Can you work these out from the model? Positions are in its coordinate system, mm. Face numbers are marked on the shaded views. A direction names the side the tool comes from. Give positions to 0.01 mm unless a question says otherwise; leave off trailing zeros. Order: outer loops, then holes, each group sorted by start corner. A loop starts at its lowest first (then second) coordinate and runs counter-clockwise, first axis right, second up. Notation, with made-up numbers: (25, -15) - (48, -15) arc R32 cw to (48, 20) - close; hole circle Ø6 at (61.25, -15). An arc over 180 degrees is marked (long way). Write each question's results on one line, items separated by ' | '. Start each with the question number.
Autodesk Fusion 360 part; units mm, degrees
sketch "Sketch1" plane through (0, 0, 0) normal (0, 1, 0) x (1, 0, 0) in component "ChargerSpacer"
  arc A0 (-5.8311, -8.732) -> (-5.8573, 8.7145) centre (0, 0) cw
  arc A1 (-4.6183, -9.4298) -> (-5.8311, -8.732) centre (-5.2363, -9.1011) cw
  line L0 (-20, 3.982) -> (0, 3.982)
  arc A2 (10.4756, 0.7154) -> (10.4777, -0.6839) centre (10.5, 0.0158) cw
  arc A3 (-4.6466, 9.4159) -> (10.4756, 0.7154) centre (0, 0) cw
  arc A4 (10.4777, -0.6839) -> (-4.6183, -9.4298) centre (0, 0) cw
  arc A5 (-5.8573, 8.7145) -> (-4.6466, 9.4159) centre (-5.2637, 9.0854) cw
  line L1 (-20, -4.0237) -> (-20, 3.982)
  circle A6 centre (0, 0) radius 8
  line L2 (0, 3.982) -> (0, -4.0237)
  line L3 (0, -4.0237) -> (-20, -4.0237)
  circle A7 centre (0, 0) radius 5
  circle A8 centre (0, 0) radius 3.75
  dimension "d8" = 10
  dimension "d9" = 7.5
extrude "Extrude8" add sketch "Sketch1" along normal blind 27 contours A0 A1 L0 A2 A3 A4 A5 A6 L3 | A0 L0 A6 L3 | L0 A6 L3 A7 | L0 A6 L3 A7 | L0 L2 L3 A7 A8 | L0 L2 L3 A7 A8 in component "ChargerSpacer"
sketch "Sketch2" plane through (0, 27, 0) normal (0, 1, 0) x (-1, 0, 0) in component "ChargerSpacer"
  circle A0 centre (0, 0) radius 4
  line L0 (6.35, 6.35) -> (-6.35, 6.35)
  line L1 (-6.35, 6.35) -> (-6.35, -6.35)
  line L2 (-6.35, -6.35) -> (6.35, -6.35)
  line L3 (6.35, -6.35) -> (6.35, 6.35)
  line L4 (6.35, 6.35) -> (-6.35, -6.35) construction
  line L5 (-6.35, 6.35) -> (6.35, -6.35) construction
  line L6 (6.35, 6.35) -> (19.35, 6.35)
  line L7 (19.35, 6.35) -> (19.35, -6.35)
  line L8 (19.35, -6.35) -> (6.35, -6.35)
  line L9 (6.35, -6.35) -> (6.35, 6.35)
  circle A1 centre (0, 0) radius 6.35
  line L10 (12.5, -3.5) -> (-12.5, -3.5)
  line L11 (-12.5, -3.5) -> (-12.5, 3.5)
  line L12 (-12.5, 3.5) -> (12.5, 3.5)
  line L13 (12.5, 3.5) -> (12.5, -3.5)
  line L14 (12.5, -3.5) -> (-12.5, 3.5) construction
  line L15 (-12.5, -3.5) -> (12.5, 3.5) construction
  arc A2 (5.8573, -8.7145) -> (5.8311, 8.732) centre (0, 0) ccw
  arc A3 (5.8311, 8.732) -> (4.6183, 9.4298) centre (5.2363, 9.1011) ccw
  arc A4 (4.6183, 9.4298) -> (-10.4777, 0.6839) centre (0, 0) ccw
  arc A5 (-10.4777, 0.6839) -> (-10.4756, -0.7154) centre (-10.5, -0.0158) ccw
  arc A6 (-10.4756, -0.7154) -> (4.6466, -9.4159) centre (0, 0) ccw
  arc A7 (4.6466, -9.4159) -> (5.8573, -8.7145) centre (5.2637, -9.0854) ccw
  circle A8 centre (0, 0) radius 3.75
  dimension "d18" = 12.7
  dimension "d19" = 12.7
  dimension "d20" = 13
  dimension "d21" = 12.7
  dimension "d22" = 12.7
  dimension "d27" = 25
  dimension "d28" = 7
extrude "Extrude9" cut sketch "Sketch1" along normal blind 4 contours L0 L2 L3 A7 A8 | L0 L2 L3 A7 A8 in component "ChargerSpacer"
extrude "Extrude10" add sketch "Sketch2" along normal blind 10 contours L0 L1 L6 L12 A2 A3 A4 | L3 L6 L9 L12 A2 | L1 L2 L8 L10 A2 A6 A7 | L3 L8 L9 L10 A2 | L1 L10 L12 A4 A5 A6 in component "ChargerSpacer"
extrude "Extrude11" cut sketch "Sketch2" against normal blind 17 contours A0 L10 L12 A8 | A0 A1 L10 L12 | A0 L12 A8 | A0 A1 L12 | A0 A1 L10 | A0 L10 A8 | A0 L10 L12 A8 | A0 A1 L10 L12 | L3 L9 A1 L12 | L3 L9 A1 L10 | L3 L9 L10 L12 A2 in component "ChargerSpacer"
fillet "Fillet1" radius 3 2 edges at (-7.5989, 10, -3.5) (-7.5989, 10, 3.5) in component "ChargerSpacer"
chamfer "Chamfer1" distance 0.5 angle 45 5 edges at (-6.35, 37, -4.925) (0, 37, -6.35) (-6.35, 37, 4.925) (0, 37, 6.35) (6.35, 37, 0) in component "ChargerSpacer"
component "ChargerSpacer" placed x (1, 0, 0) y (0, 1, 0) z (0, 0, 1) at (0, 0, 0)
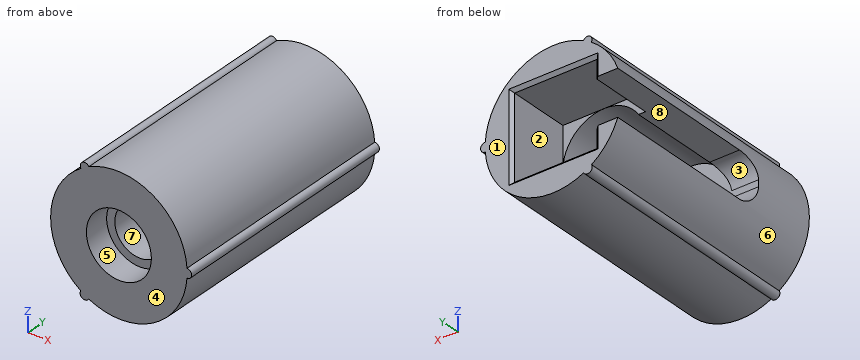
Q1. If we section it at B-B (y = 4.5): Please give me the cut outline in (x, z).
Q2. Thinking about a two-plate mould opening in X: for the marked faces 6, 7 and 8, which applies, released by +X, released by -X, zero draft, split by the parting line, or undercut?
Q3. If I drill on probe 1 along Z at (x, y) = (0, 7.8); probe 2 along Z at (x, y) = (0, 3.15); probe 3 along Y at (x, z) = (-1.5, 5.25), over which ranges is the centre line in solid material (lowest first)? Write a range as from..to.
Q4. If we section it at C-C (y = 21.5): Please give me the cut outline in (x, z).
Q5. If we section it at D-D (x = -8.75): Please give me the cut outline in (y, z).
Q6. Which directions (+Z, -Z, +X, -X, +Y, -Y) give clear straight access to the entire face, cutting with the end or side of a thin tool? Please do the marked faces 1, 2, 3, 4 and 5.
Q7. If we section it at A-A (z = -2): Please give me the cut outline in (x, y), plus the area to 3 significant figures.
Q8. Will these pins go through, and if not, where does the flat tip stop? P1, Ø3, axis at x = -4.5, z = -5, coming from the +Y side; P2, Ø0.9, axis at y = 33, z = -5, coming from the +X side; P3, Ø2, axis at x = 9, y = 30.5, coming from the +Z side; P4, Ø7.5, axis at x = -0.5, y = 31, coming from the +Z side.
Findings below:
1) outline: (-5.86, -8.71) arc R0.7 ccw (long way) to (-4.65, -9.42) arc R10.5 ccw to (10.48, -0.72) arc R0.7 ccw (long way) to (10.48, 0.68) arc R10.5 ccw to (-4.62, 9.43) arc R0.7 ccw (long way) to (-5.83, 8.73) arc R10.5 ccw to start; hole circle Ø7.5 at (0, 0)
2) face 6: released by -X | face 7: undercut | face 8: zero draft
3) probe 1: z = -10.5..-3.75, 3.75..10.5 | probe 2: z = -10.5..-5, 5..10.5 | probe 3: y = 0..10
4) outline: (-9.9, -3.5) arc R10.5 ccw to (-5.86, -8.71) arc R0.7 ccw (long way) to (-4.65, -9.42) arc R10.5 ccw to (10.48, -0.72) arc R0.7 ccw (long way) to (10.48, 0.68) arc R10.5 ccw to (-4.62, 9.43) arc R0.7 ccw (long way) to (-5.83, 8.73) arc R10.5 ccw to (-9.9, 3.5) - (-5.3, 3.5) arc R6.35 cw (long way) to (-5.3, -3.5) - close
5) outline: (0, -5.8) - (37, -5.8) - (37, -3.5) - (13, -3.5) arc R3 cw to (10, -0.5) - (10, 0.5) arc R3 cw to (13, 3.5) - (37, 3.5) - (37, 5.8) - (0, 5.8) - close
6) face 1: +Z, -Z, +X, -X, +Y | face 2: +Y | face 3: -X, +Y | face 4: +Z, -Z, +X, -X, -Y | face 5: -Y
7) outline: (-10.31, 0) - (-4.58, 0) - (-4.58, 4) - (-3.17, 4) - (-3.17, 10) - (-6.03, 10) - (-6.03, 10.4) - (-10.31, 10.4) - close; (3.17, 4) - (4.58, 4) - (4.58, 0) - (10.31, 0) - (10.31, 37) - (6.85, 37) - (6.35, 36.5) - (6.35, 27) - (6.03, 27) - (6.03, 10) - (3.17, 10) - close | area: 245 mm2
8) P1: stops at y = 36.65 | P2: stops at x = 9.46 | P3: stops at z = 6.8 | P4: stops at z = 10.5
